from build123d import *

# Parameters (mm, degrees)
SKETCH2_R             = 1.4732
BOSS_EXTRUDE1_DEPTH   = 10
FILLET2_R             = 3.175
CIRPATTERN2_START     = -49.5
CIRPATTERN2_OUTLINE_R = 1.4732
CIRPATTERN2_DEPTH     = 10


# Read off the part's stored shape, not the designer's step: CirPattern2
with BuildPart() as part:
    # Sketch1 → Revolve1 (revolve)
    with BuildSketch(Plane.YZ, mode=Mode.PRIVATE) as revolve1_sk:
        with BuildLine():
            ThreePointArc((-57.15, -39.5), (-43.428307314, -36.322800112), (-31.106422396, -29.5))
            Line((-31.106422396, -29.5), (-25.4, -29.5))
            Line((-25.4, -29.5), (-25.4, 2))
            Line((-25.4, 2), (-127, 10.888848214))
            Line((-127, 10.888848214), (-127, 8.881208539))
            Line((-127, 8.881208539), (-27.4, 0.167337652))
            Line((-27.4, 0.167337652), (-27.4, -23.683734158))
            ThreePointArc((-27.4, -23.683734158), (-41.079585236, -33.165904784), (-57.15, -37.5))
            Line((-57.15, -37.5), (-88.9, -37.5))
            Line((-88.9, -37.5), (-88.9, -82.5))
            Line((-88.9, -82.5), (-86.9, -82.5))
            Line((-86.9, -82.5), (-86.9, -39.5))
            Line((-86.9, -39.5), (-57.15, -39.5))
        make_face()
    revolve(revolve1_sk.sketch.rotate(Axis((0, 0, 14.051954895), (0, 0, -1)), 270), axis=Axis((0, 0, 14.051954895), (0, 0, -1)))

    # Sketch2 → Boss-Extrude1 (add)
    with BuildSketch(Plane(origin=(0, 0, -39.5), x_dir=(1, 0, 0), z_dir=(0, 0, -1))):
        with BuildLine():
            ThreePointArc((0, 57.15), (4, 57.009845641), (7.980380842, 56.590069991))
            ThreePointArc((7.980380842, 56.590069991), (29.37299875, 67.623432921), (53.425964916, 68.536678303))
            ThreePointArc((53.425964916, 68.536678303), (48.554411409, 72.069959989), (43.45, 75.257607589))
            ThreePointArc((43.45, 75.257607589), (19.913921564, 70.549566075), (0, 57.15))
        make_face()
        with Locations(Location((24.420129862, 69.15558596, 0), (0, 0, 180))):
            Circle(SKETCH2_R, mode=Mode.SUBTRACT)
    extrude(amount=BOSS_EXTRUDE1_DEPTH)

    # Fillet2
    fillet2_edges = [part.edges().sort_by_distance(p)[0] for p in [
        (53.425964916, -68.536678303, -44.5),
        (43.45, -75.257607589, -44.5),
    ]]
    fillet(fillet2_edges, radius=FILLET2_R)

    # CirPattern2 outline → CirPattern2 (add)
    # profile 1 of 11: a face of its own
    with BuildSketch(Plane.XY.offset(CIRPATTERN2_START)):
        with BuildLine():
            ThreePointArc((-21.383822454, -52.998628635), (-25.040821205, -51.371974591), (-28.575, -49.493351826))
            ThreePointArc((-28.575, -49.493351826), (-21.167907198, -66.538128805), (-8.985215302, -80.572781069))
            ThreePointArc((-8.985215302, -80.572781069), (-8.137140536, -84.282460346), (-11.457600483, -86.141357031))
            ThreePointArc((-11.457600483, -86.141357031), (0.680533064, -86.897335257), (12.805337694, -85.951342785))
            ThreePointArc((12.805337694, -85.951342785), (12.005662981, -85.968616711), (11.227047319, -85.785489194))
            ThreePointArc((11.227047319, -85.785489194), (-8.665120108, -72.959538869), (-21.383822454, -52.998628635))
        make_face()
        with Locations((-13.429340156, -72.100559186)):
            Circle(CIRPATTERN2_OUTLINE_R, mode=Mode.SUBTRACT)
    # profile 2 of 11: a face of its own
    with BuildSketch(Plane.XY.offset(CIRPATTERN2_START)):
        with BuildLine():
            ThreePointArc((-52.9932516, -68.871803264), (-42.859308707, -75.595566386), (-31.885923645, -80.838715188))
            ThreePointArc((-31.885923645, -80.838715188), (-32.587099225, -80.45383749), (-33.169836409, -79.905936578))
            ThreePointArc((-33.169836409, -79.905936578), (-43.983983575, -58.852254055), (-45.018247793, -35.206247537))
            ThreePointArc((-45.018247793, -35.206247537), (-47.371974591, -31.969024436), (-49.493351826, -28.575))
            ThreePointArc((-49.493351826, -28.575), (-51.601009781, -47.039756266), (-48.067815244, -65.285467609))
            ThreePointArc((-48.067815244, -65.285467609), (-49.188200591, -68.922181485), (-52.9932516, -68.871803264))
        make_face()
        with Locations((-47.680429324, -55.726245805)):
            Circle(CIRPATTERN2_OUTLINE_R, mode=Mode.SUBTRACT)
    # profile 3 of 11: a face of its own
    with BuildSketch(Plane.XY.offset(CIRPATTERN2_START)):
        with BuildLine():
            ThreePointArc((65.285467609, -48.067815244), (68.922181485, -49.188200591), (68.871803264, -52.9932516))
            ThreePointArc((68.871803264, -52.9932516), (75.595566386, -42.859308707), (80.838715188, -31.885923645))
            ThreePointArc((80.838715188, -31.885923645), (80.45383749, -32.587099225), (79.905936578, -33.169836409))
            ThreePointArc((79.905936578, -33.169836409), (58.852254055, -43.983983575), (35.206247537, -45.018247793))
            ThreePointArc((35.206247537, -45.018247793), (31.969024436, -47.371974591), (28.575, -49.493351826))
            ThreePointArc((28.575, -49.493351826), (47.039756266, -51.601009781), (65.285467609, -48.067815244))
        make_face()
        with Locations((55.726245805, -47.680429324)):
            Circle(CIRPATTERN2_OUTLINE_R, mode=Mode.SUBTRACT)
    # profile 4 of 11: a face of its own
    with BuildSketch(Plane.XY.offset(CIRPATTERN2_START)):
        with BuildLine():
            ThreePointArc((-80.329403747, -33.148105431), (-74.915033322, -44.03802655), (-68.033377494, -54.06541914))
            ThreePointArc((-68.033377494, -54.06541914), (-68.448174509, -53.381517486), (-68.678889259, -52.615652785))
            ThreePointArc((-68.678889259, -52.615652785), (-67.517374163, -28.975555294), (-56.590069991, -7.980380842))
            ThreePointArc((-56.590069991, -7.980380842), (-57.009845641, -4), (-57.15, 0))
            ThreePointArc((-57.15, 0), (-68.207663464, -14.937119024), (-74.27068291, -32.504965825))
            ThreePointArc((-74.27068291, -32.504965825), (-77.059322021, -35.094259755), (-80.329403747, -33.148105431))
        make_face()
        with Locations((-69.15558596, -24.420129862)):
            Circle(CIRPATTERN2_OUTLINE_R, mode=Mode.SUBTRACT)
    # profile 5 of 11: a face of its own
    with BuildSketch(Plane.XY.offset(CIRPATTERN2_START)):
        with BuildLine():
            ThreePointArc((80.572781069, -8.985215302), (84.282460346, -8.137140536), (86.141357031, -11.457600483))
            ThreePointArc((86.141357031, -11.457600483), (86.897335257, 0.680533064), (85.951342785, 12.805337694))
            ThreePointArc((85.951342785, 12.805337694), (85.968616711, 12.005662981), (85.785489194, 11.227047319))
            ThreePointArc((85.785489194, 11.227047319), (72.959538869, -8.665120108), (52.998628635, -21.383822454))
            ThreePointArc((52.998628635, -21.383822454), (51.371974591, -25.040821205), (49.493351826, -28.575))
            ThreePointArc((49.493351826, -28.575), (66.538128805, -21.167907198), (80.572781069, -8.985215302))
        make_face()
        with Locations((72.100559186, -13.429340156)):
            Circle(CIRPATTERN2_OUTLINE_R, mode=Mode.SUBTRACT)
    # profile 6 of 11: a face of its own
    with BuildSketch(Plane.XY.offset(CIRPATTERN2_START)):
        with BuildLine():
            ThreePointArc((-86.141357031, 11.457600483), (-86.897335257, -0.680533064), (-85.951342785, -12.805337694))
            ThreePointArc((-85.951342785, -12.805337694), (-85.968616711, -12.005662981), (-85.785489194, -11.227047319))
            ThreePointArc((-85.785489194, -11.227047319), (-72.959538869, 8.665120108), (-52.998628635, 21.383822454))
            ThreePointArc((-52.998628635, 21.383822454), (-51.371974591, 25.040821205), (-49.493351826, 28.575))
            ThreePointArc((-49.493351826, 28.575), (-66.538128805, 21.167907198), (-80.572781069, 8.985215302))
            ThreePointArc((-80.572781069, 8.985215302), (-84.282460346, 8.137140536), (-86.141357031, 11.457600483))
        make_face()
        with Locations((-72.100559186, 13.429340156)):
            Circle(CIRPATTERN2_OUTLINE_R, mode=Mode.SUBTRACT)
    # profile 7 of 11: a face of its own
    with BuildSketch(Plane.XY.offset(CIRPATTERN2_START)):
        with BuildLine():
            ThreePointArc((74.27068291, 32.504965825), (77.059322021, 35.094259755), (80.329403747, 33.148105431))
            ThreePointArc((80.329403747, 33.148105431), (74.915033322, 44.03802655), (68.033377494, 54.06541914))
            ThreePointArc((68.033377494, 54.06541914), (68.448174509, 53.381517486), (68.678889259, 52.615652785))
            ThreePointArc((68.678889259, 52.615652785), (67.517374163, 28.975555294), (56.590069991, 7.980380842))
            ThreePointArc((56.590069991, 7.980380842), (57.009845641, 4), (57.15, 0))
            ThreePointArc((57.15, 0), (68.207663464, 14.937119024), (74.27068291, 32.504965825))
        make_face()
        with Locations((69.15558596, 24.420129862)):
            Circle(CIRPATTERN2_OUTLINE_R, mode=Mode.SUBTRACT)
    # profile 8 of 11: a face of its own
    with BuildSketch(Plane.XY.offset(CIRPATTERN2_START)):
        with BuildLine():
            ThreePointArc((-68.871803264, 52.9932516), (-75.595566386, 42.859308707), (-80.838715188, 31.885923645))
            ThreePointArc((-80.838715188, 31.885923645), (-80.45383749, 32.587099225), (-79.905936578, 33.169836409))
            ThreePointArc((-79.905936578, 33.169836409), (-58.852254055, 43.983983575), (-35.206247537, 45.018247793))
            ThreePointArc((-35.206247537, 45.018247793), (-31.969024436, 47.371974591), (-28.575, 49.493351826))
            ThreePointArc((-28.575, 49.493351826), (-47.039756266, 51.601009781), (-65.285467609, 48.067815244))
            ThreePointArc((-65.285467609, 48.067815244), (-68.922181485, 49.188200591), (-68.871803264, 52.9932516))
        make_face()
        with Locations((-55.726245805, 47.680429324)):
            Circle(CIRPATTERN2_OUTLINE_R, mode=Mode.SUBTRACT)
    # profile 9 of 11: a face of its own
    with BuildSketch(Plane.XY.offset(CIRPATTERN2_START)):
        with BuildLine():
            ThreePointArc((48.067815244, 65.285467609), (49.188200591, 68.922181485), (52.9932516, 68.871803264))
            ThreePointArc((52.9932516, 68.871803264), (42.859308707, 75.595566386), (31.885923645, 80.838715188))
            ThreePointArc((31.885923645, 80.838715188), (32.587099225, 80.45383749), (33.169836409, 79.905936578))
            ThreePointArc((33.169836409, 79.905936578), (43.983983575, 58.852254055), (45.018247793, 35.206247537))
            ThreePointArc((45.018247793, 35.206247537), (47.371974591, 31.969024436), (49.493351826, 28.575))
            ThreePointArc((49.493351826, 28.575), (51.601009781, 47.039756266), (48.067815244, 65.285467609))
        make_face()
        with Locations((47.680429324, 55.726245805)):
            Circle(CIRPATTERN2_OUTLINE_R, mode=Mode.SUBTRACT)
    # profile 10 of 11: a face of its own
    with BuildSketch(Plane.XY.offset(CIRPATTERN2_START)):
        with BuildLine():
            ThreePointArc((-33.148105431, 80.329403747), (-44.03802655, 74.915033322), (-54.06541914, 68.033377494))
            ThreePointArc((-54.06541914, 68.033377494), (-53.381517486, 68.448174509), (-52.615652785, 68.678889259))
            ThreePointArc((-52.615652785, 68.678889259), (-28.975555294, 67.517374163), (-7.980380842, 56.590069991))
            ThreePointArc((-7.980380842, 56.590069991), (-4, 57.009845641), (0, 57.15))
            ThreePointArc((0, 57.15), (-14.937119024, 68.207663464), (-32.504965825, 74.27068291))
            ThreePointArc((-32.504965825, 74.27068291), (-35.094259755, 77.059322021), (-33.148105431, 80.329403747))
        make_face()
        with Locations((-24.420129862, 69.15558596)):
            Circle(CIRPATTERN2_OUTLINE_R, mode=Mode.SUBTRACT)
    # profile 11 of 11: a face of its own
    with BuildSketch(Plane.XY.offset(CIRPATTERN2_START)):
        with BuildLine():
            ThreePointArc((8.985215302, 80.572781069), (8.137140536, 84.282460346), (11.457600483, 86.141357031))
            ThreePointArc((11.457600483, 86.141357031), (-0.680533064, 86.897335257), (-12.805337694, 85.951342785))
            ThreePointArc((-12.805337694, 85.951342785), (-12.005662981, 85.968616711), (-11.227047319, 85.785489194))
            ThreePointArc((-11.227047319, 85.785489194), (8.665120108, 72.959538869), (21.383822454, 52.998628635))
            ThreePointArc((21.383822454, 52.998628635), (25.040821205, 51.371974591), (28.575, 49.493351826))
            ThreePointArc((28.575, 49.493351826), (21.167907198, 66.538128805), (8.985215302, 80.572781069))
        make_face()
        with Locations((13.429340156, 72.100559186)):
            Circle(CIRPATTERN2_OUTLINE_R, mode=Mode.SUBTRACT)
    extrude(amount=CIRPATTERN2_DEPTH)


solid = part.part
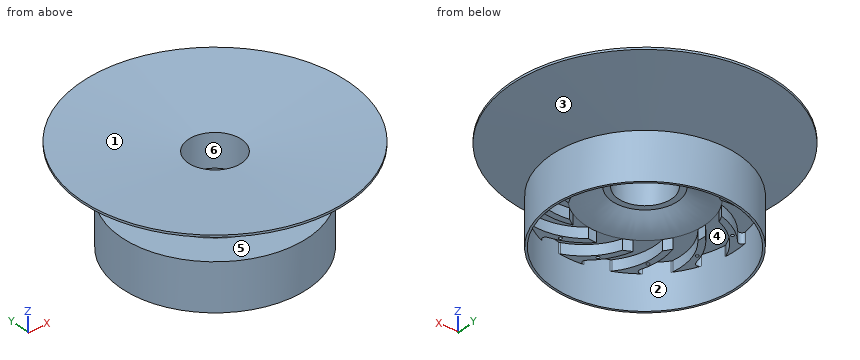
Here's how the part is built. I have some questions about the finished solid (model axes, mm). Face numbers are marked on the shaded views. A direction names the side the tool comes from. Round coordinates to 2 decimals unless told otherwise and drop trailing zeros. Loops run counter-clockwise (first coordinate to the right, second up) from the corner with the lowest first, then second, coordinate; pieces in that order, holes last. Notation, with made-up numbers: (-9.75, 27.5) -> (-1.75, 27.5) arc R31 ccw to (-1.75, 66.5) -> close; hole circle Ø5 at (88, 11). An arc over 180 degrees is marked (long way). Write each question's results on one line, items separated by ' | '.
(1) If I drill on L1, parallel to Z at x = 19, y = -48; L2, parallel to X at y = -56, z = -43.5; L3, parallel to Z at x = 71.5, y = -18.5, over which ranges is the centre line in solid material (lowest first)?
Worked answers:
L1: -38.7 to -36.67, 2.29 to 4.29 | L2: -69.04 to -66.45, -50.59 to -49.13, -46.23 to -44.66, -26.47 to -20.18, 66.45 to 69.04 | L3: -39.5 to -37.5, 4.23 to 6.24
(2) If we section it at B-B, the plane z = -55: List the corners of the cut face in (x, y) for me.
Worked answers:
outline: circle Ø177.8 at (0, 0); hole circle Ø173.8 at (0, 0)
(3) For the marked faces 1, 2 and 3, which set-ups out of +Z, -Z, +X, -X, +Y, -Y let a thin tool reach every point of the face, with its end or its side?
Worked answers:
face 1: +Z | face 2: -Z | face 3: none
(4) If we section it at A-A, the plane z = -17.5: List the corners of the cut face in (x, y) for me, then the cut area to 3 significant figures.
Worked answers:
outline: circle Ø54.8 at (0, 0); hole circle Ø50.8 at (0, 0) | area: 332 mm2
(5) We'd pull the mould along Z, two halves only. Please class the marked faces 4, 5 and 6: released by +Z, released by -Z, zero draft, split by the parting line, or undercut.
Worked answers:
face 4: released by -Z | face 5: undercut | face 6: zero draft
(6) For P1, Ø17, axis at x = -42.5, y = 44, coming from the -Z side; P2, Ø6.5, axis at x = 42, y = -63.5, coming from the -Z side; P3, Ø4, axis at x = -84.5, y = -56, coming from the -Z side, each with a flat end and sliding along its axis, tell me the tip position at first contact or that it passes through.
Worked answers:
P1: z = -49.5 | P2: z = -39.5 | P3: z = 6.46
